Work out the finished part from the listing and answer in its coordinate system (mm). Round coordinates to 2 decimals unless told otherwise and drop trailing zeros. Order: outer loops, then holes, each group sorted by start corner. A loop starts at its lowest first (then second) coordinate and runs counter-clockwise, first axis right, second up. Notation, with made-up numbers: M 39,69 L 87,69 A27 cw 87,96 Z; hole C -18.5,-31 d7. An arc over 180 degrees is marked long. Return JSON: item names as keys, results as strings.
from build123d import *

# Parameters (mm, degrees)
SKETCH1_R           = 1.5
BOSS_EXTRUDE1_DEPTH = 3
SKETCH2_R           = 2.5
CUT_EXTRUDE1_DEPTH  = 3


with BuildPart() as part:
    # Sketch1 → Boss-Extrude1 (new body)
    with BuildSketch(Plane(origin=(0, 0, 0), x_dir=(1, 0, 0), z_dir=(0, 1, 0))):
        with BuildLine():
            Line((-4.930066486, 60.833333333), (-14.790199458, 2.5))
            ThreePointArc((-14.790199458, 2.5), (0, -15), (14.790199458, 2.5))
            Line((14.790199458, 2.5), (4.930066486, 60.833333333))
            ThreePointArc((4.930066486, 60.833333333), (0, 65), (-4.930066486, 60.833333333))
        make_face()
        with Locations((0, 60)):
            Circle(SKETCH1_R, mode=Mode.SUBTRACT)
    extrude(amount=BOSS_EXTRUDE1_DEPTH)

    # Sketch2 → Cut-Extrude1 (cut)
    with BuildSketch(Plane(origin=(0, 3, 0), x_dir=(1, 0, 0), z_dir=(0, 1, 0))):
        Circle(SKETCH2_R)
    extrude(amount=-CUT_EXTRUDE1_DEPTH, mode=Mode.SUBTRACT)


solid = part.part
Item 1: Find section A-A (z = 0). Determine the outline of the cut face in (x, y).
Output:
{"outline": "M -15,0 L -2.5,0 L -2.5,3 L -15,3 Z; M 2.5,0 L 15,0 L 15,3 L 2.5,3 Z"}
Item 2: The mould has two halves that part along X. Classify faces 1 (the flat face through (0, 3, -17)), 2 (the cylindrical face through (-0.54, 1.52, 2.44)), 3 (the flat face through (9.93, 1.48, -31.26)): pulls with the +X half, pulls with the -X half, needs draft (parallel to the pull), parting line crosses it, or undercut.
Output:
{"face 1": "needs draft", "face 2": "undercut", "face 3": "pulls with the +X half"}
Item 3: Find section C-C (y = 1.25). Determine the outline of the cut face in (x, z).
Output:
{"outline": "M -14.79,-2.5 L -4.93,-60.83 A5 ccw 4.93,-60.83 L 14.79,-2.5 A15 ccw long Z; hole C 0,0 d5; hole C 0,-60 d3"}
Item 4: Find section B-B (x = 0). Determine the outline of the cut face in (y, z), plus the area to 3 significant figures.
Output:
{"outline": "M 0,-65 L 3,-65 L 3,-61.5 L 0,-61.5 Z; M 0,-58.5 L 3,-58.5 L 3,-2.5 L 0,-2.5 Z; M 0,2.5 L 3,2.5 L 3,15 L 0,15 Z", "area": "216 mm^2"}
Item 5: This flat-tipped pin is pushed along its axis until it touches: pin 1 (1 mm diameter, centred on y = 2, z = -53.5, fed in from +X). Where does it stop, or does it pass through?
Output:
{"pin 1": "stops at x = 6.25"}
Item 6: Find section D-D (z = -60). Determine the outline of the cut face in (x, y), plus the area to 3 significant figures.
Output:
{"outline": "M -5.07,0 L -1.5,0 L -1.5,3 L -5.07,3 Z; M 1.5,0 L 5.07,0 L 5.07,3 L 1.5,3 Z", "area": "21.4 mm^2"}
Item 7: Consider line 1 along X through (y, z) = (1.55, 0); line 2 along X through (y, z) = (1.55, -60); line 3 along X through (y, z) = (0.7, -22.5). Determine where each line is inside the solid, lowest interval first. Write a range as [from, to].
Output:
{"line 1": "x = [-15, -2.5], [2.5, 15]", "line 2": "x = [-5.07, -1.5], [1.5, 5.07]", "line 3": "x = [-11.41, 11.41]"}
